Autodesk Inventor part; units mm, degrees
ref_plane "YZ Plane" through (0, 0, 0) normal (1, 0, 0) x (0, 1, 0)
ref_plane "XZ Plane" through (0, 0, 0) normal (0, 1, 0) x (-1, 0, 0)
ref_plane "XY Plane" through (0, 0, 0) normal (0, 0, 1) x (1, 0, 0)
sketch "Sketch3" plane through (0, 0, 0) normal (0, 0, 1) x (1, 0, 0)
  circle A0 centre (0, 0) radius 11.5
  circle A1 centre (0, 0) radius 4
  circle A2 centre (7, 0) radius 1.5
  circle A3 centre (3.5, 6.0622) radius 1.5
  circle A4 centre (-3.5, 6.0622) radius 1.5
  circle A5 centre (-7, 0) radius 1.5
  circle A6 centre (-3.5, -6.0622) radius 1.5
  circle A7 centre (3.5, -6.0622) radius 1.5
  dimension "d0" = 23
  dimension "d1" = 8
  dimension "d4" = 3
  dimension "d5" = 7
  dimension "d12" = 360
extrude "Extrusion1" add sketch "Sketch3" along normal blind 5 contours A0 | A3 | A5 | A7
sketch "Sketch4" plane through (0, 0, 0) normal (1, 0, 0) x (0, 1, 0)
  line L0 (-11.5, 0) -> (11.5, 0)
  line L1 (-4, 5) -> (4, 5)
  line L2 (4, 0) -> (-4, 0)
  circle A0 centre (0, 2.5) radius 1.5
  line L3 (4, 0) -> (4, 5)
  point P0 (0, 0)
  point P1 (0, 0)
  point P2 (4, 2.5)
  dimension "d14" = 3
extrude "Extrusion2" cut sketch "Sketch4" against normal through all
thread "Thread1"
thread "Thread2"
thread "Thread3"
thread "Thread4"
equation "\"d15\" = d14"
properties part number "6mm Mounting Hub, thin" material "Aluminum 6061"
Can you work these out from the model? Positions are in its coordinate system, mm. A direction names the side the tool comes from. Coordinates: 2 decimals unless noted, no trailing zeros. Order: outer loops, then holes, each group sorted by start corner. A loop starts at its lowest first (then second) coordinate and runs counter-clockwise, first axis right, second up. Notation, with made-up numbers: (56, 18.25) - (87, 18.25) arc R23 cw to (87, 29.25) - close; hole circle Ø2 at (69, 6.25). An arc over 180 degrees is marked (long way). Answer as a JSON object with one key per item and string values. Group by question number.
Q1. Imagine slicing it at C-C (z = 2.15). Please give me the cut outline in (x, y).
Q2. I need wall thicknesses on line 1 (Y direction, x = -3.5, z = 3.05); line 2 (Y direction, x = -6.5, z = 2.5); line 3 (X direction, y = 5.5, z = 1.9). Which ranges of each line are inside material? Lowest first, please. Write a range as from..to.
Q3. On a 3-axis mill with a long thin cutter (end or side, diameter ignored), from which of +Z, -Z, +X, -X, +Y, -Y can I reach the whole of each face in a straight line? I mean faces 4 (the face through (-8, 0, 1)), 5 (the face through (0, -5, 0)). Say none if no direction works.
Q4. Imagine slicing it at A-A (x = 0). Please give me the cut outline in (y, z), and give its area (3 significant figures).
Q5. Imagine slicing it at B-B (y = -2.75). Please give me the cut outline in (x, z).
Q6. Will these pins go through, and if not, where does the flat tip stop? P1, Ø3, axis at y = 3, z = 4, coming from the +X side; P2, Ø2.5, axis at x = -3.5, y = -6.06, coming from the +Z side; P3, Ø1, axis at x = -5, z = 4, coming from the -Y side.
Q7. Imagine slicing it at D-D (y = 0). Please give me the cut outline in (x, z).
Q8. We'd pull the mould along X, two halves only. Please class faces 1 (the face through (0, -5, 5)), 2 (the face through (-2.1, 6.6, 2.5)), 3 (the face through (10.97, -3.45, 2.46)): +X half, -X half, draft (parallel to the pull), parting line (faces both ways), or undercut.
Determined:
{
 "1": {"outline": "(-11.41, -1.46) arc R11.5 ccw (long way) to (-11.41, 1.46) - (-3.72, 1.46) arc R4 cw (long way) to (-3.72, -1.46) - close; hole circle Ø3 at (-3.5, -6.06); hole circle Ø3 at (-3.5, 6.06); hole circle Ø3 at (7, 0)"},
 "2": {"line 1": "y = -10.95..-7.56, -4.56..-1.94, 1.94..4.56, 7.56..10.95", "line 2": "y = -9.49..-1.5, 1.5..9.49", "line 3": "x = -10.1..-4.89, -2.11..10.1"},
 "3": {"face 4": "-X", "face 5": "-Z, +X, -X, +Y, -Y"},
 "4": {"outline": "(-11.5, 0) - (-4, 0) - (-4, 5) - (-11.5, 5) - close; (4, 0) - (11.5, 0) - (11.5, 5) - (4, 5) - close", "area": "75.0 mm2"},
 "5": {"outline": "(-11.17, 0) - (-2.9, 0) - (-2.9, 5) - (-11.17, 5) - close; (2.9, 0) - (11.17, 0) - (11.17, 5) - (2.9, 5) - close"},
 "6": {"P1": "stops at x = 11.4", "P2": "passes through", "P3": "stops at y = -10.58"},
 "7": {"outline": "(-11.5, 0) - (-4, 0) - (-4, 1) - (-11.5, 1) - close; (-11.5, 4) - (-4, 4) - (-4, 5) - (-11.5, 5) - close; (4, 0) - (5.5, 0) - (5.5, 5) - (4, 5) - close; (8.5, 0) - (11.5, 0) - (11.5, 5) - (8.5, 5) - close"},
 "8": {"face 1": "draft", "face 2": "undercut", "face 3": "parting line"}
}
